Source: CAD feature listing. Evaluate the final solid. Frame: model axes, mm. Face numbers are marked on the shaded views. Round coordinates to 2 decimals unless told otherwise and drop trailing zeros. Order: outer loops, then holes, each group sorted by start corner. A loop starts at its lowest first (then second) coordinate and runs counter-clockwise, first axis right, second up.
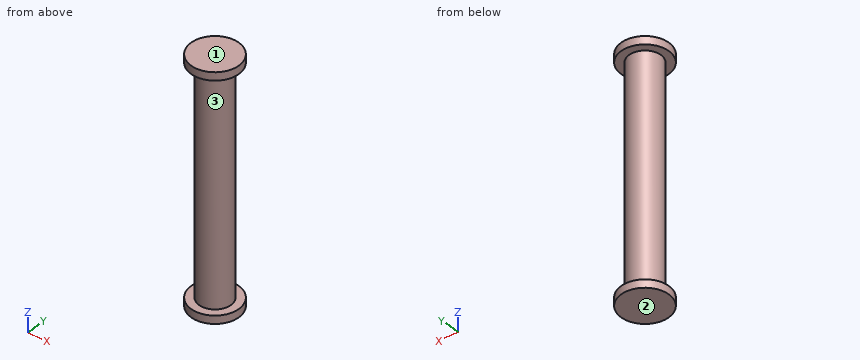
```python
from build123d import *

# Parameters (mm, degrees)
SKETCH1_R           = 4.95
BOSS_EXTRUDE1_DEPTH = 70
SKETCH2_R           = 7.45
BOSS_EXTRUDE2_DEPTH = 2.5
SKETCH3_R           = 7.45
BOSS_EXTRUDE3_DEPTH = 2.5


with BuildPart() as part:
    # Sketch1 → Boss-Extrude1 (new body)
    with BuildSketch(Plane.XY):
        Circle(SKETCH1_R)
    extrude(amount=BOSS_EXTRUDE1_DEPTH)

    # Sketch2 → Boss-Extrude2 (add)
    with BuildSketch(Plane(origin=(0, 0, 0), x_dir=(-1, 0, 0), z_dir=(0, 0, -1))):
        Circle(SKETCH2_R)
    extrude(amount=BOSS_EXTRUDE2_DEPTH)

    # Sketch3 → Boss-Extrude3 (add)
    with BuildSketch(Plane.XY.offset(70)):
        Circle(SKETCH3_R)
    extrude(amount=BOSS_EXTRUDE3_DEPTH)


solid = part.part
```
1. Section B-B on x = 0. Return loops of the section in (y, z), plus the area to 4 significant figures.
2. Pull-direction query (Z, two-part tool) for the marked faces 1, 2 and 3; classes: released by +Z, released by -Z, zero draft, split by the parting line, or undercut.
3. Section A-A on y = 6.5. Return loops of the section in (x, z).
4. First-contact query: pin 1 (2 mm diameter, centred on x = -5, z = 36, fed in from +Y); pin 2 (1.5 mm diameter, centred on y = 0.5, z = 60, fed in from -X); pin 3 (8 mm diameter, centred on x = -1.5, z = 31.5, fed in from +Y). Flat tips, straight axial feed; report the tip coordinate or a pass-through.
5. Section D-D on z = 5. Return loops of the section in (x, y), plus the area to 3 significant figures.
6. Line query: line 1 along Z through (x, y) = (-4, 3.5); line 2 along X through (y, z) = (-0.25, 26); line 3 along X through (y, z) = (-3, 50.5). Output: solid intervals per line, ascending.
Result:
1. outline: (-7.45, -2.5) - (7.45, -2.5) - (7.45, 0) - (4.95, 0) - (4.95, 70) - (7.45, 70) - (7.45, 72.5) - (-7.45, 72.5) - (-7.45, 70) - (-4.95, 70) - (-4.95, 0) - (-7.45, 0) - close
1. area: 767.5 mm2
2. face 1: released by +Z
2. face 2: released by -Z
2. face 3: undercut
3. outline: (-3.64, -2.5) - (3.64, -2.5) - (3.64, 0) - (-3.64, 0) - close; (-3.64, 70) - (3.64, 70) - (3.64, 72.5) - (-3.64, 72.5) - close
4. pin 1: stops at y = 2.92
4. pin 2: stops at x = -4.95
4. pin 3: stops at y = 4.95
5. outline: circle Ø9.9 at (0, 0)
5. area: 77.0 mm2
6. line 1: z = -2.5 to 0, 70 to 72.5
6. line 2: x = -4.94 to 4.94
6. line 3: x = -3.94 to 3.94
